Design review of the part built by this model. Coordinates are the model's own, in mm. A direction names the side the tool comes from. Coordinates: 2 decimals unless noted, no trailing zeros. Write each loop counter-clockwise with the first axis right and the second up, starting at its lowest first coordinate (ties: lowest second). Pieces come first, ordered by that corner, then holes.
Autodesk Inventor part; units mm, degrees
ref_plane "YZ Plane" through (0, 0, 0) normal (1, 0, 0) x (0, 1, 0)
ref_plane "XZ Plane" through (0, 0, 0) normal (0, 1, 0) x (-1, 0, 0)
ref_plane "XY Plane" through (0, 0, 0) normal (0, 0, 1) x (1, 0, 0)
sketch "Sketch1" plane through (0, 0, 0) normal (0, 0, 1) x (1, 0, 0)
  line L0 (0, 0) -> (152.4, 0)
  line L1 (152.4, 0) -> (152.4, 152.4)
  line L2 (152.4, 152.4) -> (0, 152.4)
  line L3 (0, 152.4) -> (0, 0)
  dimension "d0" = 152.4
  dimension "d1" = 152.4
extrude "Extrusion1" add sketch "Sketch1" along normal blind 45.339
sketch "Sketch2" plane through (0, 0, 45.339) normal (0, 0, 1) x (1, 0, 0)
  line L0 (0, 0) -> (152.4, 0)
  line L1 (0, 152.4) -> (0, 0)
  circle A0 centre (76.2, 76.2) radius 6.35
  circle A1 centre (76.2, 76.2) radius 9.017
  dimension "d13" = 12.7
  dimension "d14" = 18.034
  dimension "d15" = 76.2
  dimension "d16" = 76.2
extrude "Extrusion2" add sketch "Sketch2" along normal blind 1.905
hole "Hole2" at (76.2, 76.2, 45.339) direction (0, 0, -1) diameter 12.7 depth 18.415
hole "Hole3" at (76.2, 76.2, 26.924) direction (0, 0, -1) diameter 12.192 depth 7.747
hole "Hole4" at (76.2, 76.2, 19.177) direction (0, 0, -1) diameter 11.684 depth 0.508
properties part number "Door"
(1) Wall thickness on line 1 (X direction, y = 76, z = 24); line 2 (X direction, y = 76.2, z = 19); line 3 (Y direction, x = 76.2, z = 24.25): over which ranges is each line inside the solid? List them lowest first.
(2) Insertion check: pin 1 Ø7.5 at (x, y) = (76.2, 76.2) entering from +Z; pin 2 Ø11.5 at (x, y) = (76.2, 76.2) entering from -Z; pin 3 Ø10 at (x, y) = (44, 49) entering from +Z. Each pin has a flat end and moves straight along its axis. Give the tip position at first contact, or say it passes through.
(3) Consider section A-A (x = 136). Give the boundary of the cut face in (y, z).
(4) For faces 1 (the cylindrical face through (67.19, 75.8, 46.28)), 2 (the flat face through (70, 74, 47.244)), list the 3-axis set-ups (+Z, -Z, +X, -X, +Y, -Y) from which the entire face can be reached by the end or side of a thin tool; tool diameter is ignored.
Results:
1. line 1: x = 0 to 70.11, 82.29 to 152.4
1. line 2: x = 0 to 70.36, 82.04 to 152.4
1. line 3: y = 0 to 70.1, 82.3 to 152.4
2. pin 1: stops at z = 18.67
2. pin 2: stops at z = 0
2. pin 3: stops at z = 45.34
3. outline: (0, 0) - (152.4, 0) - (152.4, 45.34) - (0, 45.34) - close
4. face 1: +Z
4. face 2: +Z, +X, -X, +Y, -Y
